Model file for the job. Use its own axes, mm. A direction names the side the tool comes from. Coordinates: 2 decimals unless noted, no trailing zeros. Order: outer loops, then holes, each group sorted by start corner. A loop starts at its lowest first (then second) coordinate and runs counter-clockwise, first axis right, second up. Notation, with made-up numbers: M -10.5,-39 L 43.5,-39 A9 cw 43.5,-31 Z; hole C 4,48.5 d10. An arc over 180 degrees is marked long. Return JSON: item names as keys, results as strings.
```python
from build123d import *

# Parameters (mm, degrees)
F1_DEPTH = 12.7


with BuildPart() as f1:
    # F0 (on Right) → F1 (new body)
    with BuildSketch(Plane.YZ):
        Polygon((0, 32.104064), (0, 0), (27.176283, 0), (27.176283, 15.24), (50.036283, 15.24), (50.036283, 0), (131.275059, 0), (131.275059, 15.24), (154.135059, 15.24), (154.135059, 0), (262.550118, 0), (0, 95.560428), (0, 54.964064), (15.24, 54.964064), (15.24, 32.104064), align=None)
    extrude(amount=F1_DEPTH)


solid = f1.part
```
Item 1: Drop flat-ended pins along their axis: pin 1 Ø1 at (x, y) = (9, 203) entering from +Z; pin 2 Ø1.5 at (x, z) = (9.5, 45) entering from -Y. Give the stop position or say it passes through.
Check result:
{"pin 1": "stops at z = 21.86", "pin 2": "stops at y = 15.24"}
Item 2: Saw through at A-A (x = 2). Write the cut outline in (y, z).
Check result:
{"outline": "M 0,0 L 27.18,0 L 27.18,15.24 L 50.04,15.24 L 50.04,0 L 131.28,0 L 131.28,15.24 L 154.14,15.24 L 154.14,0 L 262.55,0 L 0,95.56 L 0,54.96 L 15.24,54.96 L 15.24,32.1 L 0,32.1 Z"}
Item 3: Saw through at C-C (z = 62.5). Write the cut outline in (x, y), and give its area (3 significant figures).
Check result:
{"outline": "M 0,0 L 12.7,0 L 12.7,90.83 L 0,90.83 Z", "area": "1,150 mm2"}
Item 4: 3-axis set-ups, long thin cutter, end or side, ignore diameter. For faces 1 (the flat face through (6, 38, 15.24)), 2 (the flat face through (6, 8, 54.964)), 3 (the flat face through (6, 90, 0)): which of +Z, -Z, +X, -X, +Y, -Y reach the whole face in a straight line?
Check result:
{"face 1": "-Z, +X, -X", "face 2": "+X, -X, -Y", "face 3": "-Z, +X, -X, +Y, -Y"}
Item 5: Wall check: line 1 (Z direction, x = 4.5, y = 14.5); line 2 (Z direction, x = 7.5, y = 97.5); line 3 (Z direction, x = 2.75, y = 210.5). Give the ranges that are in metal, low to high.
Check result:
{"line 1": "z = 0 to 32.1, 54.96 to 90.28", "line 2": "z = 0 to 60.07", "line 3": "z = 0 to 18.94"}
Item 6: Saw through at B-B (y = 110.5). Write the cut outline in (x, z).
Check result:
{"outline": "M 0,0 L 12.7,0 L 12.7,55.34 L 0,55.34 Z"}
Item 7: Pull direction Y, two halves, no side cores. Call faces 4 (the flat face through (6, 50.036, 8)), 5 (the flat face through (6, 13, 0)), 6 (the flat face through (6, 15.24, 44)), 7 (the flat face through (6, 143, 15.24)): +Y half, -Y half, draft (parallel to the pull), parting line (faces both ways), or undercut.
Check result:
{"face 4": "undercut", "face 5": "draft", "face 6": "-Y half", "face 7": "undercut"}
